Check sheet for the drawn part. Datum: minimum x, y, z corner. Units: mm. Round coordinates to 2 decimals unless told otherwise and drop trailing zeros. Write each loop counter-clockwise with the first axis right and the second up, starting at its lowest first coordinate (ties: lowest second). Pieces come first, ordered by that corner, then holes. Notation, with made-up numbers: (5.5, -31) - (34.5, -31) arc R12 cw to (34.5, -20) - close; hole circle Ø7 at (-25.75, -13.5). An arc over 180 degrees is marked (long way). Answer as a JSON object with one key per item and string values. Group by question number.
Item 1: Thickness scan on line 1 (Y direction, x = 1.25, z = 10); line 2 (Z direction, x = 0.15, y = 63); line 3 (Y direction, x = 0.95, z = 3.5). Record the ranges inside material, lowest first.
Item 2: Sectioned sample at B-B on x = 0.8. Count the separate pieces of the cut face and the enclosed holes in it, plus the area to 3 significant figures.
Item 3: Sectioned sample at D-D on z = 2. Record the boundary of the cut face in (x, y) (1 decimal), plus the area to 3 significant figures.
Item 4: Sectioned sample at C-C on y = 112.5. Record the boundary of the cut face in (x, z).
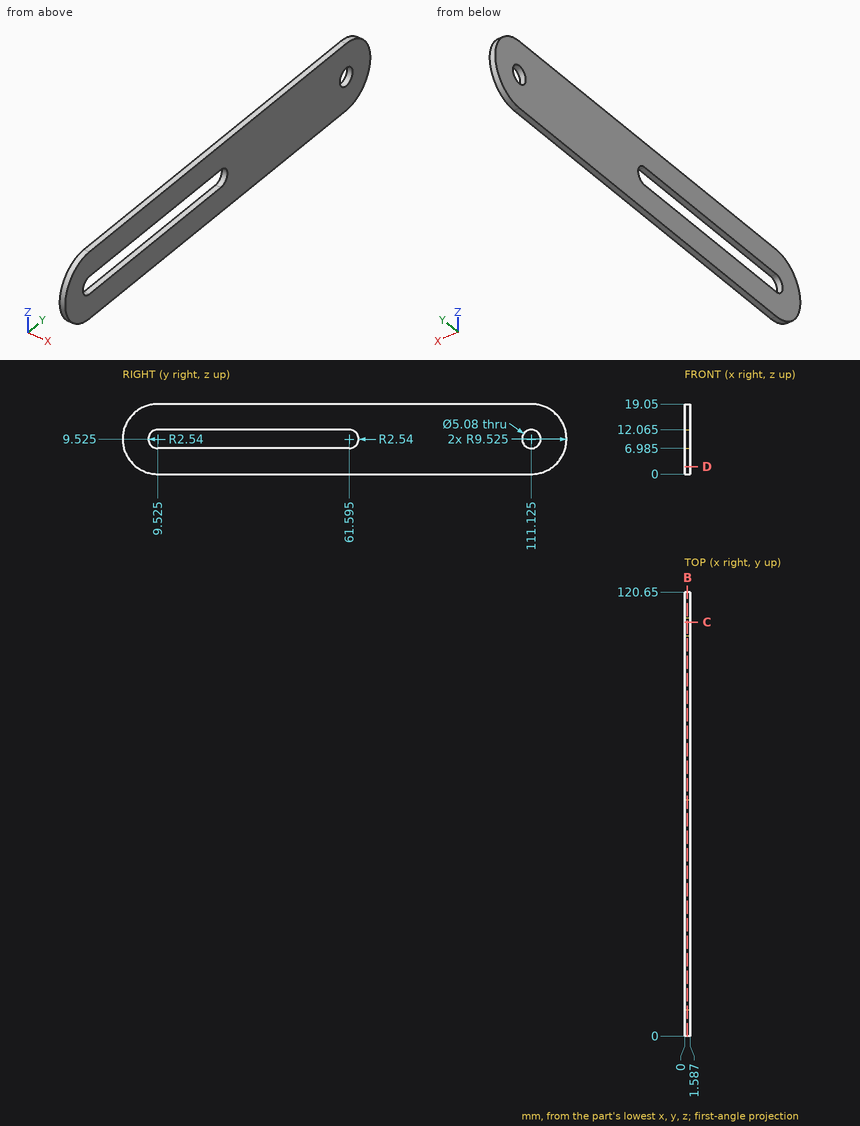
Completed:
{
 "1": {"line 1": "0.01 to 7.03, 64.09 to 108.63, 113.62 to 120.64", "line 2": "0 to 7.41, 11.64 to 19.05", "line 3": "2.15 to 118.5"},
 "2": {"separate pieces": "1", "enclosed holes": "2", "area": "1,920 mm²"},
 "3": {"outline": "(0, 3.7) - (1.6, 3.7) - (1.6, 117) - (0, 117) - close", "area": "180 mm²"},
 "4": {"outline": "(0, 0.1) - (1.59, 0.1) - (1.59, 7.39) - (0, 7.39) - close; (0, 11.66) - (1.59, 11.66) - (1.59, 18.95) - (0, 18.95) - close"}
}
